Geometry check sheet. Reference: the model listing, model coordinates, mm. Face numbers are marked on the shaded views. A direction names the side the tool comes from. Round coordinates to 2 decimals unless told otherwise and drop trailing zeros. Write each loop counter-clockwise with the first axis right and the second up, starting at its lowest first coordinate (ties: lowest second). Pieces come first, ordered by that corner, then holes.
Item 1: Cross-section at C-C (x = -1). Enter the section's corners in (y, z), then the cut area to 3 significant figures.
Item 2: Access from +Z, -Z, +X, -X, +Y, -Y to the whole of each face (thin tool, end or side, straight path). Record for the marked faces 4, 5, 6 and 7.
Item 3: Cross-section at D-D (z = -7). Enter the section's corners in (x, y) (3 decimals), then the cut area to 3 significant figures.
Item 4: Scan lines: probe 1 along X at (y, z) = (3.5, 0); probe 2 along Y at (x, z) = (50.25, 0); probe 3 along Z at (x, y) = (35, 31). Record each from-to range of solid material in increasing order.
Item 5: Cross-section at B-B (x = 28.5). Enter the section's corners in (y, z).
Item 6: Depth check by flat-ended pin: P1, Ø12, axis at x = -7.5, z = -0.5, coming from the +Y side; P2, Ø3, axis at x = 37, y = 8.5, coming from the -Z side; P3, Ø1.3, axis at x = 28, z = 17, coming from the -Y side. Enter the tip coordinate at first touch or a pass-through.
Item 7: Draft check along Z on the marked faces 1, 2 and 3. Enter one of: pulls with the +Z half, pulls with the -Z half, needs draft (parallel to the pull), parting line crosses it, or undercut.
Item 8: Cross-section at A-A (z = 1). Enter the section's corners in (x, y).
from build123d import *
from build123d.topology import SkipClean

# Parameters (mm, degrees)
EXTRUDE_1_DEPTH      = 30
EXTRUDE_START        = -40
EXTRUDE_5_DEPTH      = 40
CUT_EXTRUDE_START    = -42
SKETCH_11_R          = 18
CUT_EXTRUDE_2_DEPTH  = 42
CUT_EXTRUDE_3_DEPTH  = 20
CUT_EXTRUDE_6_DEPTH  = 30
EXTRUDE_7_DEPTH      = 5
EXTRUDE_7_DEPTH_BACK = 10
SKETCH_14_R          = 0.75
SKETCH_14_W          = 41
SKETCH_14_H          = 21
EXTRUDE_9_DEPTH      = 2
SKETCH_18_R          = 20.85
CUT_EXTRUDE_8_DEPTH  = 20
CUT_EXTRUDE_START_2  = -38
CUT_EXTRUDE_10_DEPTH = 38
EXTRUDE_10_DEPTH     = 5
EXTRUDE_11_DEPTH     = 2
SKETCH_22_R          = 18.25
SKETCH_22_R_2        = 15.25
EXTRUDE_13_DEPTH     = 8
SKETCH_29_R          = 1.7
CUT_EXTRUDE_13_DEPTH = 73.622310708
SKETCH_30_R          = 2.75
CUT_EXTRUDE_14_DEPTH = 30


# Read off the part's stored shape, not the designer's step: 凸台-拉伸5
with BuildPart() as part:
    # 草图1 → 凸台-拉伸1 (new body)
    with BuildSketch(Plane(origin=(0, 0, 0), x_dir=(1, 0, 0), z_dir=(0, 1, 0))):
        with BuildLine():
            Line((40, 12.5), (12.951833847, 12.5))
            ThreePointArc((12.951833847, 12.5), (-18, 0), (12.951833847, -12.5))
            Line((12.951833847, -12.5), (40, -12.5))
            Line((40, -12.5), (40, -14.5))
            Line((40, -14.5), (13.774977314, -14.5))
            ThreePointArc((13.774977314, -14.5), (-20, 0), (13.774977314, 14.5))
            Line((13.774977314, 14.5), (40, 14.5))
            Line((40, 14.5), (40, 12.5))
        make_face()
    extrude(amount=EXTRUDE_1_DEPTH)

    # 凸台-拉伸5 outline → 凸台-拉伸5 (add)
    with BuildSketch(Plane(origin=(40, 0, 0), x_dir=(0, 0, -1), z_dir=(1, 0, 0)).offset(EXTRUDE_START)):
        with BuildLine():
            ThreePointArc((14.5, 9.225022686), (0, 43), (-14.5, 9.225022686))
            ThreePointArc((-14.5, 9.225022686), (0, 3), (14.5, 9.225022686))
        make_face()
        with BuildLine():
            ThreePointArc((14.5, 12.334635496), (0, 5), (-14.5, 12.334635496))
            ThreePointArc((-14.5, 12.334635496), (0, 41), (14.5, 12.334635496))
        make_face(mode=Mode.SUBTRACT)
    extrude(amount=EXTRUDE_5_DEPTH)

    # 草图11 → 切除-拉伸2 (cut)
    with BuildSketch(Plane(origin=(40, 0, 0), x_dir=(0, 0, -1), z_dir=(1, 0, 0)).offset(CUT_EXTRUDE_START)):
        with Locations((0, 23)):
            Circle(SKETCH_11_R)
    extrude(amount=CUT_EXTRUDE_2_DEPTH, mode=Mode.SUBTRACT)

    # 草图10 → 切除-拉伸3 (cut)
    with BuildSketch(Plane(origin=(0, 30, 0), x_dir=(1, 0, 0), z_dir=(0, 1, 0))):
        with BuildLine():
            Line((0, 20), (40, 20))
            Line((40, 20), (40, -20))
            Line((40, -20), (0, -20))
            ThreePointArc((0, -20), (-20, 0), (0, 20))
        make_face()
    extrude(amount=CUT_EXTRUDE_3_DEPTH, mode=Mode.SUBTRACT)

    # 草图13 → 切除-拉伸6 (cut)
    with SkipClean():  # the faces are left unmerged after this step: merging them gives an invalid solid
        with BuildSketch(Plane.XZ):
            with BuildLine():
                Line((40, -12.5), (12.951833847, -12.5))
                ThreePointArc((12.951833847, -12.5), (-18, 0), (12.951833847, 12.5))
                Line((12.951833847, 12.5), (40, 12.5))
                Line((40, 12.5), (40, -12.5))
            make_face()
        extrude(amount=-CUT_EXTRUDE_6_DEPTH, mode=Mode.SUBTRACT)

    # 草图15 → 凸台-拉伸7 (add, two sides: drawn at the far end of the back side and taken through both)
    with SkipClean():  # the faces are left unmerged after this step: merging them gives an invalid solid
        with BuildSketch(Plane(origin=(40, 0, 0), x_dir=(0, 0, -1), z_dir=(1, 0, 0)).offset(-EXTRUDE_7_DEPTH_BACK)):
            with BuildLine():
                Line((12.5, 10.048166153), (12.5, 7.387505004))
                ThreePointArc((12.5, 7.387505004), (0, 43), (-12.5, 7.387505004))
                Line((-12.5, 7.387505004), (-12.5, 10.048166153))
                ThreePointArc((-12.5, 10.048166153), (0, 41), (12.5, 10.048166153))
            make_face()
        extrude(amount=EXTRUDE_7_DEPTH + EXTRUDE_7_DEPTH_BACK)

    # 草图14 → 凸台-拉伸9 (add)
    # profile 1 of 2: a face of its own
    with SkipClean():  # the faces are left unmerged after this step: merging them gives an invalid solid
        with BuildSketch(Plane(origin=(0, 30, 0), x_dir=(1, 0, 0), z_dir=(0, 1, 0))):
            with BuildLine():
                Line((7, -18.734993995), (30, -18.734993995))
                Line((30, -18.734993995), (30, -16.583123952))
                Line((30, -16.583123952), (7, -16.583123952))
                ThreePointArc((7, -16.583123952), (-18, 0), (7, 16.583123952))
                Line((7, 16.583123952), (30, 16.583123952))
                Line((30, 16.583123952), (30, 18.734993995))
                Line((30, 18.734993995), (7, 18.734993995))
                ThreePointArc((7, 18.734993995), (-20, 0), (7, -18.734993995))
            make_face()
        # profile 2 of 2: a face of its own
        with BuildSketch(Plane(origin=(0, 30, 0), x_dir=(1, 0, 0), z_dir=(0, 1, 0))):
            with BuildLine():
                Line((40, 16.583123952), (40, -16.583123952))
                Line((40, -16.583123952), (7, -16.583123952))
                ThreePointArc((7, -16.583123952), (-18, 0), (7, 16.583123952))
                Line((7, 16.583123952), (40, 16.583123952))
            make_face()
            with Locations(Location((-13.5, 5.25, 0), (0, 0, 270))):
                Circle(SKETCH_14_R, mode=Mode.SUBTRACT)
            with Locations(Location((-13.5, -5.25, 0), (0, 0, 270))):
                Circle(SKETCH_14_R, mode=Mode.SUBTRACT)
            with Locations(Location((35.5, 5.25, 0), (0, 0, 270))):
                Circle(SKETCH_14_R, mode=Mode.SUBTRACT)
            with Locations(Location((35.5, -5.25, 0), (0, 0, 270))):
                Circle(SKETCH_14_R, mode=Mode.SUBTRACT)
            with Locations((11, 0)):
                Rectangle(SKETCH_14_W, SKETCH_14_H, mode=Mode.SUBTRACT)
        extrude(amount=EXTRUDE_9_DEPTH)

    # 草图18 → 切除-拉伸8 (cut)
    with SkipClean():  # the faces are left unmerged after this step: merging them gives an invalid solid
        with BuildSketch(Plane(origin=(0, 32, 0), x_dir=(1, 0, 0), z_dir=(0, 1, 0))):
            with Locations((20.85, 0)):
                Circle(SKETCH_18_R)
        extrude(amount=CUT_EXTRUDE_8_DEPTH, mode=Mode.SUBTRACT)

    # 草图19 → 切除-拉伸10 (cut)
    with SkipClean():  # the faces are left unmerged after this step: merging them gives an invalid solid
        with BuildSketch(Plane(origin=(45, 0, 0), x_dir=(0, 0, -1), z_dir=(1, 0, 0)).offset(CUT_EXTRUDE_START_2)):
            with BuildLine():
                Line((-17.860571099, 32), (-18.734993995, 32))
                Line((-18.734993995, 32), (-18.734993995, 30))
                ThreePointArc((-18.734993995, 30), (-18.325087889, 31.011938208), (-17.860571099, 32))
            make_face()
            with BuildLine():
                Line((18.734993995, 32), (17.860571099, 32))
                ThreePointArc((17.860571099, 32), (18.325087889, 31.011938208), (18.734993995, 30))
                Line((18.734993995, 30), (18.734993995, 32))
            make_face()
        extrude(amount=CUT_EXTRUDE_10_DEPTH, mode=Mode.SUBTRACT)

    # 草图20 → 凸台-拉伸10 (add)
    with SkipClean():  # the faces are left unmerged after this step: merging them gives an invalid solid
        with BuildSketch(Plane(origin=(40, 0, 0), x_dir=(0, 0, -1), z_dir=(1, 0, 0))):
            with BuildLine():
                Line((-14.5, 9.225022686), (-14.5, 0))
                Line((-14.5, 0), (-12.5, 0))
                Line((-12.5, 0), (-12.5, 7.387505004))
                ThreePointArc((-12.5, 7.387505004), (-13.531227506, 8.27227505), (-14.5, 9.225022686))
            make_face()
            with BuildLine():
                Line((12.5, 7.387505004), (12.5, 0))
                Line((12.5, 0), (14.5, 0))
                Line((14.5, 0), (14.5, 9.225022686))
                ThreePointArc((14.5, 9.225022686), (13.531227506, 8.27227505), (12.5, 7.387505004))
            make_face()
            with BuildLine():
                Line((-16.583123952, 30), (16.583123952, 30))
                ThreePointArc((16.583123952, 30), (16.11684397, 31.015443871), (15.588457268, 32))
                Line((15.588457268, 32), (-15.588457268, 32))
                ThreePointArc((-15.588457268, 32), (-16.11684397, 31.015443871), (-16.583123952, 30))
            make_face()
        extrude(amount=EXTRUDE_10_DEPTH)

    # 草图21 → 凸台-拉伸11 (add)
    with SkipClean():  # the faces are left unmerged after this step: merging them gives an invalid solid
        with BuildSketch(Plane(origin=(45, 0, 0), x_dir=(0, 0, -1), z_dir=(1, 0, 0))):
            with BuildLine():
                Line((-14.5, 0), (14.5, 0))
                Line((14.5, 0), (14.5, 9.225022686))
                ThreePointArc((14.5, 9.225022686), (0, 43), (-14.5, 9.225022686))
                Line((-14.5, 9.225022686), (-14.5, 0))
            make_face()
        extrude(amount=EXTRUDE_11_DEPTH)

    # 草图22 → 凸台-拉伸13 (add)
    with SkipClean():  # the faces are left unmerged after this step: merging them gives an invalid solid
        with BuildSketch(Plane(origin=(47, 0, 0), x_dir=(0, 0, -1), z_dir=(1, 0, 0))):
            with Locations((0, 23)):
                Circle(SKETCH_22_R)
            with Locations((0, 23)):
                Circle(SKETCH_22_R_2, mode=Mode.SUBTRACT)
        extrude(amount=EXTRUDE_13_DEPTH)

    # 草图29 → 切除-拉伸13 (cut, through all)
    with SkipClean():  # the faces are left unmerged after this step: merging them gives an invalid solid
        with BuildSketch(Plane.XZ):
            with Locations(Location((-6.5, -15.5, 0), (0, 0, 90))):
                Circle(SKETCH_29_R)
            with Locations(Location((28.5, -15.5, 0), (0, 0, 90))):
                Circle(SKETCH_29_R)
            with Locations(Location((28.5, 15.5, 0), (0, 0, 90))):
                Circle(SKETCH_29_R)
            with Locations(Location((-6.5, 15.5, 0), (0, 0, 90))):
                Circle(SKETCH_29_R)
        extrude(amount=-CUT_EXTRUDE_13_DEPTH, mode=Mode.SUBTRACT)

    # 草图30 → 切除-拉伸14 (cut)
    with SkipClean():  # the faces are left unmerged after this step: merging them gives an invalid solid
        with BuildSketch(Plane.XZ):
            with Locations((-6.5, -15.5)):
                Circle(SKETCH_30_R)
            with Locations(Location((28.5, -15.5, 0), (0, 0, 203.195097041))):
                Circle(SKETCH_30_R)
            with Locations(Location((28.5, 15.5, 0), (0, 0, 338.676313737))):
                Circle(SKETCH_30_R)
            with Locations((-6.5, 15.5)):
                Circle(SKETCH_30_R)
        extrude(amount=-CUT_EXTRUDE_14_DEPTH, mode=Mode.SUBTRACT)


solid = part.part
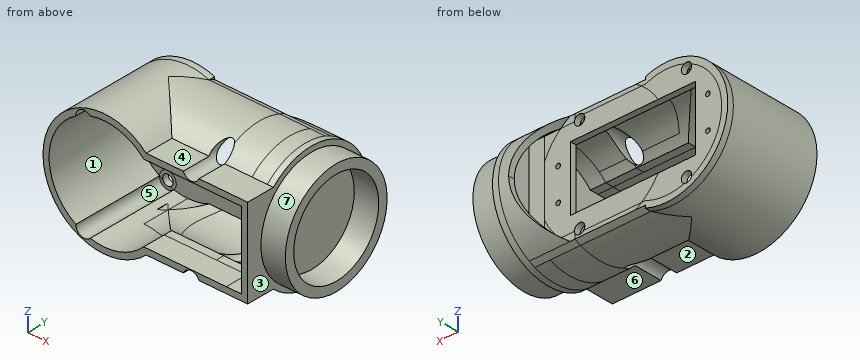
Resolved:
1. outline: (0, -19.97) - (32, -19.97) - (32, -10.5) - (30, -10.5) - (30, -17.97) - (24, -17.97) arc R18 cw to (22, -17.97) - (0, -17.97) - close; (0, 17.97) - (22, 17.97) arc R18 cw to (24, 17.97) - (30, 17.97) - (30, 10.5) - (32, 10.5) - (32, 19.97) - (0, 19.97) - close
1. area: 158 mm2
2. face 4: +Z, +X, -Y
2. face 5: -Y
2. face 6: -Z, +X, -Y
2. face 7: +X
3. outline: (-18.735, 0) - (-16.583, 0) - (-16.583, 30) - (-9.5, 30) - (-9.5, 32) - (-18.735, 32) - close; (31.5, 30) - (45, 30) - (45, 0) - (47, 0) - (47, 6.146) - (55, 6.146) - (55, 9.451) - (47, 9.451) - (47, 36.549) - (55, 36.549) - (55, 39.854) - (47, 39.854) - (47, 41.735) - (40.49, 41.735) - (40.49, 39.583) - (45, 39.583) - (45, 32) - (31.5, 32) - close
3. area: 256 mm2
4. probe 1: x = -20 to -18, 45 to 47
4. probe 2: y = 4.75 to 7.75, 38.25 to 41.25
4. probe 3: z = -18.33 to -5.81, -4.69 to 4.69, 5.81 to 18.33
5. outline: (0, -12.75) - (10.29, -12.75) arc R18 cw to (10.05, -12.5) - (0, -12.5) - close; (0, 12.5) - (10.05, 12.5) arc R18 cw to (10.29, 12.75) - (0, 12.75) - close; (14.82, -18.25) arc R20 ccw to (32, -17.86) - (32, -17.2) - (30, -17.2) - (30, -18.25) - close; (14.82, 18.25) - (30, 18.25) - (30, 17.2) - (32, 17.2) - (32, 17.86) arc R20 ccw to start; (30, -13.8) - (32, -13.8) - (32, -10.5) - (30, -10.5) - close; (30, 10.5) - (32, 10.5) - (32, 13.8) - (30, 13.8) - close
6. P1: stops at y = 32
6. P2: stops at z = -15.2
6. P3: stops at y = 30
7. face 1: undercut
7. face 2: pulls with the -Z half
7. face 3: needs draft
8. outline: (-19.97, 0) - (-17.97, 0) - (-17.97, 30) - (-9.5, 30) - (-9.5, 32) - (-19.97, 32) - close; (31.5, 30) - (45, 30) - (45, 0) - (47, 0) - (47, 4.78) - (55, 4.78) - (55, 7.78) - (47, 7.78) - (47, 38.22) - (55, 38.22) - (55, 41.22) - (47, 41.22) - (47, 42.97) - (41.68, 42.97) - (41.68, 40.97) - (45, 40.97) - (45, 32) - (31.5, 32) - close
